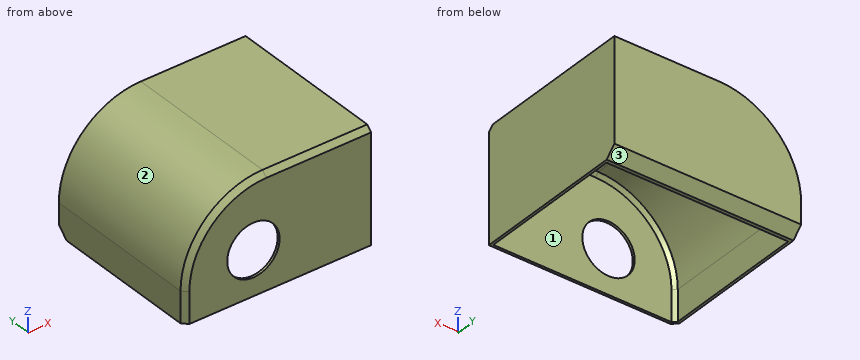
```python
from build123d import *

# Parameters (mm, degrees)
F0_W     = 187.050685
F0_H     = 162.711885
F1_DEPTH = 113
F2_R     = 82.083261
F3_SIZE  = 5
F4_SIZE  = 10
F5_T     = -2.5
F6_R     = 26.235681
F7_DEPTH = 78


with BuildPart() as f1:
    # F0 (on Top) → F1 (new body)
    with BuildSketch(Plane.XY):
        with Locations((-0.18569, -41.488969)):
            Rectangle(F0_W, F0_H)
    extrude(amount=F1_DEPTH)

    # F2
    f2_edges = [f1.edges().sort_by_distance(p)[0] for p in [
        (-93.711033, -41.48897, 113),
    ]]
    fillet(f2_edges, radius=F2_R)

    # F3
    f3_edges = [f1.edges().sort_by_distance(p)[0] for p in [
        (40.85594, -122.844912, 113),
    ]]
    chamfer(f3_edges, length=F3_SIZE)

    # F4
    f4_edges = [f1.edges().sort_by_distance(p)[0] for p in [
        (-0.185691, 39.866973, 0),
    ]]
    chamfer(f4_edges, length=F4_SIZE)

    # F5
    f5_openings = [f1.faces().sort_by_distance(p)[0] for p in [
        (-0.145476, -46.456271, 0),
    ]]
    offset(amount=F5_T, openings=f5_openings)

    # F6 (on face) → F7 (cut)
    with BuildSketch(Plane.XZ.offset(122.844912)):
        with Locations((-24.566162, 44.215515)):
            Circle(F6_R)
    extrude(amount=-F7_DEPTH, mode=Mode.SUBTRACT)


solid = f1.part
```
Source: CAD feature listing. Evaluate the final solid. Frame: model axes, mm. Face numbers are marked on the shaded views. Round coordinates to 2 decimals unless told otherwise and drop trailing zeros. Order: outer loops, then holes, each group sorted by start corner. A loop starts at its lowest first (then second) coordinate and runs counter-clockwise, first axis right, second up. Notation, with made-up numbers: (56, 70.25) -> (79, 70.25) arc R23 cw to (79, 85.25) -> close; hole circle Ø10 at (-13, -0.75). An arc over 180 degrees is marked (long way). Use CSV: the item, a comma, the result in double quotes.
(1) Section C-C on z = 21.5. Return the cut outline in (x, y), and give its area (3 significant figures).
Report:
outline,"(-93.71, -117.84) -> (-88.71, -122.84) -> (-37.69, -122.84) -> (-37.69, -120.34) -> (-87.68, -120.34) -> (-91.21, -116.81) -> (-91.21, 37.37) -> (90.84, 37.37) -> (90.84, -120.34) -> (-11.44, -120.34) -> (-11.44, -122.84) -> (93.34, -122.84) -> (93.34, 39.87) -> (-93.71, 39.87) -> close"
area,"1,650 mm^2"
(2) Ray query, L1, parallel to Y at x = -39.5, z = 93; L2, parallel to X at y = -83.5, z = 16; L3, parallel to Z at x = -8, y = -16. Return the intervals inside material, ascending.
Report:
L1,"-122.84 to -120.34, 37.37 to 39.87"
L2,"-93.71 to -91.21, 90.84 to 93.34"
L3,"110.5 to 113"
(3) First-contact query: pin 1 Ø6 at (x, z) = (-35, 30) entering from -Y; pin 2 Ø4 at (y, z) = (-83, 83) entering from -X; pin 3 Ø1.5 at (y, z) = (-44.5, 95.5) entering from -X. Flat tips, straight axial feed; report the tip coordinate or a pass-through.
Report:
pin 1,"y = 37.37"
pin 2,"x = -76.66"
pin 3,"x = -63.23"
(4) Section A-A on x = 18. Return the cut outline in (y, z).
Report:
outline,"(-122.84, 0) -> (-120.34, 0) -> (-120.34, 106.96) -> (-116.81, 110.5) -> (37.37, 110.5) -> (37.37, 11.04) -> (26.33, 0) -> (29.87, 0) -> (39.87, 10) -> (39.87, 113) -> (-117.84, 113) -> (-122.84, 108) -> close"
(5) Section B-B on y = 12. Return the cut outline in (x, z).
Report:
outline,"(-93.71, 0) -> (-91.21, 0) -> (-91.21, 30.92) arc R79.58 cw to (-11.63, 110.5) -> (90.84, 110.5) -> (90.84, 0) -> (93.34, 0) -> (93.34, 113) -> (-11.63, 113) arc R82.08 ccw to (-93.71, 30.92) -> close"
(6) Pull-direction query (Y, two-part tool) for the marked faces 1, 2 and 3; classes: +Y half, -Y half, draft (parallel to the pull), parting line (faces both ways), or undercut.
Report:
face 1,"undercut"
face 2,"draft"
face 3,"+Y half"
